Could you check a few things on this model? Use its own coordinates, in mm. Round coordinates to 2 decimals unless told otherwise and drop trailing zeros. Write each loop counter-clockwise with the first axis right and the second up, starting at its lowest first coordinate (ties: lowest second). Pieces come first, ordered by that corner, then holes. Notation, with made-up numbers: (80, 80) - (129, 80) arc R12 cw to (129, 92) - close; hole circle Ø1 at (53, 35.25). An arc over 180 degrees is marked (long way). Write each question's results on one line, items separated by ' | '. Start each with the question number.
(1) Imagine slicing it at A-A on y = -16.5. Write out the boundary of the cut face in (x, z), then the cut area to 3 significant figures.
(2) Imagine slicing it at C-C on y = 3. Write out the boundary of the cut face in (x, z).
(3) Imagine slicing it at B-B on x = 4. Write out the boundary of the cut face in (y, z).
(4) Please list where these lines run through material, in increasing order: line 1 (X direction, y = -17.5, z = 17); line 2 (X direction, y = 9, z = 1.5); line 3 (Z direction, x = 64, y = -10). Write a range as [from, to].
(5) For P1, Ø4, axis at y = -16.5, z = 15.45, coming from the -X side; P2, Ø1.5, axis at x = 24.5, y = -8.5, coming from the +Z side; P3, Ø1.5, axis at y = 13.5, z = 1, coming from the -X side; P4, Ø4.5, axis at x = -86.5, z = 8.5, coming from the +Y side, each with a flat end and sliding along its axis, tell me the tip position at first contact or that it passes through.
```python
from build123d import *

# Parameters (mm, degrees)
SKETCH1_W           = 173
SKETCH1_H           = 43
BOSS_EXTRUDE1_DEPTH = 3
SKETCH2_R           = 5
SKETCH2_W           = 13
SKETCH2_H           = 10
BOSS_EXTRUDE2_DEPTH = 2
BOSS_EXTRUDE3_START = 2
SKETCH3_R           = 5
SKETCH3_W           = 13
SKETCH3_H           = 10
BOSS_EXTRUDE3_DEPTH = 2
SKETCH4_R           = 1.5
CUT_EXTRUDE1_DEPTH  = 200
FILLET1_R           = 10
FILLET2_R           = 2


with BuildPart() as part:
    # Sketch1 → Boss-Extrude1 (new body)
    with BuildSketch(Plane.XY):
        Rectangle(SKETCH1_W, SKETCH1_H)
    extrude(amount=BOSS_EXTRUDE1_DEPTH)

    # Sketch2 → Boss-Extrude2 (add)
    with BuildSketch(Plane.ZY.offset(86.5)):
        with Locations((13, -16.5)):
            Circle(SKETCH2_R)
        with Locations((6.5, -16.5)):
            Rectangle(SKETCH2_W, SKETCH2_H)
    extrude(amount=BOSS_EXTRUDE2_DEPTH)

    # Sketch3 → Boss-Extrude3 (add)
    with BuildSketch(Plane(origin=(86.5, 0, 0), x_dir=(0, 0, -1), z_dir=(1, 0, 0)).offset(BOSS_EXTRUDE3_START)):
        with Locations((-13, -16.5)):
            Circle(SKETCH3_R)
        with Locations((-6.5, -16.5)):
            Rectangle(SKETCH3_W, SKETCH3_H)
    extrude(amount=-BOSS_EXTRUDE3_DEPTH)

    # Sketch4 → Cut-Extrude1 (cut)
    with BuildSketch(Plane(origin=(88.5, 0, 0), x_dir=(0, 0, -1), z_dir=(1, 0, 0))):
        with Locations((-15.446473159, -16.5)):
            Circle(SKETCH4_R)
    extrude(amount=-CUT_EXTRUDE1_DEPTH, mode=Mode.SUBTRACT)

    # Fillet1
    # the kernel refuses this fillet: 10 mm, written as the material it adds along each edge
    with BuildSketch(Plane(origin=(-86.5, -11.5, 3), x_dir=(0, 1, 0), z_dir=(0, 0, -1))) as fillet1_piece_1:
        with BuildLine():
            CenterArc((6, -10), FILLET1_R, 90, 36.869897646)
            Line((0, -2), (0, 0))
            Line((0, 0), (6, 0))
        make_face()
    extrude(amount=3)
    with BuildSketch(Plane(origin=(86.5, -11.5, 3), x_dir=(0, 1, 0), z_dir=(0, 0, -1))) as fillet1_piece_2:
        with BuildLine():
            CenterArc((6, 10), FILLET1_R, 233.130102354, 36.869897646)
            Line((0, 2), (0, 0))
            Line((0, 0), (6, 0))
        make_face()
    extrude(amount=3)

    # Fillet2
    fillet2_edges = [part.edges().sort_by_distance(p)[0] for p in [
        (-86.5, -16.5, 3),
        (86.5, -16.5, 3),
    ]]
    fillet(fillet2_edges, radius=FILLET2_R)


solid = part.part
```
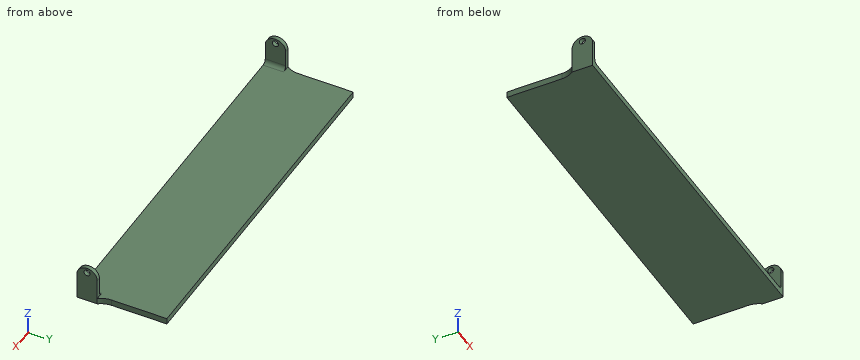
Response:
1) outline: (-88.5, 0) - (88.5, 0) - (88.5, 13.95) - (86.5, 13.95) - (86.5, 5) arc R2 cw to (84.5, 3) - (-84.5, 3) arc R2 cw to (-86.5, 5) - (-86.5, 13.95) - (-88.5, 13.95) - close; (-88.5, 16.95) - (-86.5, 16.95) - (-86.5, 18) - (-88.5, 18) - close; (86.5, 16.95) - (88.5, 16.95) - (88.5, 18) - (86.5, 18) - close | area: 581 mm²
2) outline: (-86.5, 0) - (86.5, 0) - (86.5, 3) - (-86.5, 3) - close
3) outline: (-21.5, 0) - (21.5, 0) - (21.5, 3) - (-21.5, 3) - close
4) line 1: [-88.5, -86.5], [86.5, 88.5] | line 2: [-86.5, 86.5] | line 3: [0, 3]
5) P1: x = -88.5 | P2: z = 3 | P3: x = -86.5 | P4: y = -11.5
